Autodesk Inventor part; units mm, degrees
ref_plane "YZ Plane" through (0, 0, 0) normal (1, 0, 0) x (0, 1, 0)
ref_plane "XZ Plane" through (0, 0, 0) normal (0, 1, 0) x (-1, 0, 0)
ref_plane "XY Plane" through (0, 0, 0) normal (0, 0, 1) x (1, 0, 0)
sketch "Sketch1" plane through (0, 0, 0) normal (0, 0, 1) x (1, 0, 0)
  line L0 (-1181.1, -609.6) -> (1181.1, -609.6)
  line L1 (1181.1, -609.6) -> (1181.1, 609.6)
  line L2 (1181.1, 609.6) -> (-1181.1, 609.6)
  line L3 (-1181.1, 609.6) -> (-1181.1, -609.6)
  line L4 (-1181.1, -609.6) -> (1181.1, 609.6) construction
  line L5 (1181.1, -609.6) -> (-1181.1, 609.6) construction
  line L6 (0, 609.6) -> (0, -609.6)
  line L7 (0, 609.6) -> (1181.1, -609.6)
  line L8 (-31.9258, 578.6719) -> (31.9258, 640.5281)
  line L9 (1149.1742, -640.5281) -> (1213.0258, -578.6719)
  line L10 (-31.9258, 578.6719) -> (1149.1742, -640.5281)
  line L11 (1213.0258, -578.6719) -> (31.9258, 640.5281)
  line L12 (-31.9258, 578.6719) -> (-61.8874, 609.6)
  line L13 (1181.1, -609.6) -> (-1181.1, 609.6) construction
  line L14 (0, 609.6) -> (-1181.1, -609.6)
  line L15 (31.9258, 578.6719) -> (-31.9258, 640.5281)
  line L16 (-1149.1742, -640.5281) -> (-1213.0258, -578.6719)
  line L17 (31.9258, 578.6719) -> (-1149.1742, -640.5281)
  line L18 (-1213.0258, -578.6719) -> (-31.9258, 640.5281)
  line L19 (31.9258, 578.6719) -> (61.8874, 609.6)
  point P0 (0, 0)
  point P1 (-1181.1, -545.7163)
  point P2 (-1119.2126, -609.6)
  point P3 (61.8874, 609.6)
  point P4 (0, 545.7163)
  point P5 (1119.2126, -609.6)
  point P6 (1181.1, -545.7163)
  point P7 (61.8874, 609.6)
  dimension "d0" = 2362.2
  dimension "d1" = 1219.2
  dimension "d3" = 88.9
  dimension "d4" = 88.9
extrude "Extrusion1" add sketch "Sketch1" along normal blind 38.1 contours L17 L7 L0 L10 | L17 L19 L11 L1 L7
properties part number "S_2x4x65.081"
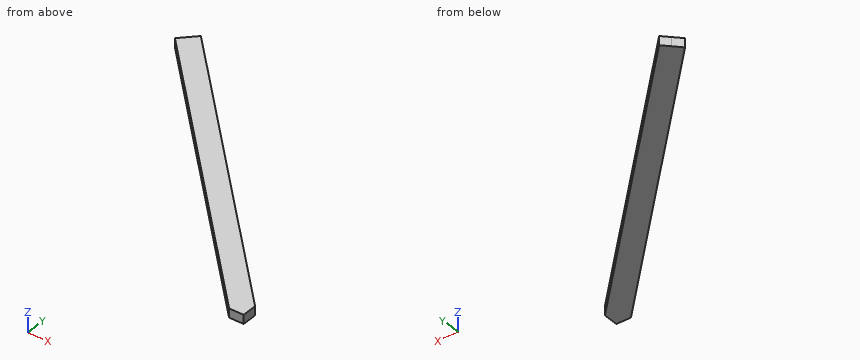
Verification items for the finished model (mm, model axes). Coordinates: 2 decimals unless noted, no trailing zeros. Loops run counter-clockwise (first coordinate to the right, second up) from the corner with the lowest first, then second, coordinate; pieces in that order, holes last. Notation, with made-up numbers: (67.25, -6) -> (101.25, -6) arc R21 cw to (101.25, 22) -> close; hole circle Ø11 at (-15, 36). An arc over 180 degrees is marked (long way). Answer as a JSON object with one key per item and string values. Group by question number.
Item 1: Sectioned sample at A-A on z = 16.5. Record the boundary of the cut face in (x, y).
Item 2: Depth check by flat-ended pin: pin 1 (5 mm diameter, centred on x = 801.5, z = 31, fed in from -Y); pin 2 (10 mm diameter, centred on y = -296, z = 7.5, fed in from +X); pin 3 (2 mm diameter, centred on x = 1005.5, z = 34, fed in from +Y). Enter the tip coordinate at first touch or a pass-through.
Item 3: Sectioned sample at B-B on x = 267. Record the boundary of the cut face in (y, z).
Item 4: Sectioned sample at C-C on y = 523. Record the boundary of the cut face in (x, z).
Item 5: Scan lines: probe 1 along X at (y, z) = (-32.5, 33); probe 2 along X at (y, z) = (92, 21); probe 3 along Y at (x, z) = (354, 8.5). Record each from-to range of solid material in increasing order.
Evaluation:
{
 "1": {"outline": "(0, 545.72) -> (1119.21, -609.6) -> (1181.1, -609.6) -> (1181.1, -545.72) -> (61.89, 609.6) -> close"},
 "2": {"pin 1": "stops at y = -284.22", "pin 2": "stops at x = 944.03", "pin 3": "stops at y = -363.42"},
 "3": {"outline": "(270.1, 0) -> (397.87, 0) -> (397.87, 38.1) -> (270.1, 38.1) -> close"},
 "4": {"outline": "(22.01, 0) -> (145.78, 0) -> (145.78, 38.1) -> (22.01, 38.1) -> close"},
 "5": {"probe 1": "x = 560.15 to 683.92", "probe 2": "x = 439.54 to 563.31", "probe 3": "y = 180.3 to 308.06"}
}
